Part model, mm, in its own coordinate system. Give positions to 0.01 mm unless a question says otherwise; leave off trailing zeros. Order: outer loops, then holes, each group sorted by start corner. A loop starts at its lowest first (then second) coordinate and runs counter-clockwise, first axis right, second up.
1. Slice it at D-D on x = 0. List the corners of the cut face in (y, z).
2. Slice it at A-A on z = -0.5. List the corners of the cut face in (x, y).
3. Probe line 1 (Z direction, x = -8, y = 4.25); line 2 (X direction, y = -1.5, z = -2.75) (3 decimals); line 3 (X direction, y = 1.75, z = -2). List the from-to ranges inside material, lowest first.
4. Slice it at B-B on z = -6. List the corners of the cut face in (x, y) (3 decimals), and give its area (3 significant figures).
5. Slice it at C-C on y = 4. List the corners of the cut face in (x, z).
6. Drop a flat-ended pin along its axis: pin 1 Ø2 at (y, z) = (4.5, -4.5) entering from +X (3 decimals). Give the stop position or say it passes through.
from build123d import *

# Parameters (mm, degrees)
SKETCH_W               = 37.5
SKETCH_H               = 12
PAD_DEPTH              = 1.4
SKETCH001_W            = 33
SKETCH001_H            = 12
PAD001_DEPTH           = 1.5
SKETCH002_W            = 0.25
SKETCH002_H            = 0.25
PAD002_DEPTH           = 1.5
PAD002_DEPTH_BACK      = 9.5
LINEARPATTERN_COUNT    = 4
LINEARPATTERN_PITCH    = 2.5
PAD003_DEPTH           = 2.25
LINEARPATTERN001_COUNT = 4
LINEARPATTERN001_PITCH = 2.5


with BuildPart() as part:
    # Sketch → Pad (new body)
    with BuildSketch(Plane.XY):
        Rectangle(SKETCH_W, SKETCH_H)
    extrude(amount=PAD_DEPTH)

    # Sketch001 (on Face6 of Pad) → Pad001 (join)
    with BuildSketch(Plane.XY.offset(1.4)):
        with Locations((2.25, 0)):
            Rectangle(SKETCH001_W, SKETCH001_H)
    extrude(amount=PAD001_DEPTH)

    # Sketch002 (on Face5 of Pad001) → Pad002 (join, two sides)
    with BuildSketch(Plane.XY.offset(1.4)) as pad002_sk:
        with Locations((-17.55, -4)):
            Rectangle(SKETCH002_W, SKETCH002_H)
    pad002 = extrude(amount=PAD002_DEPTH) + extrude(pad002_sk.sketch, amount=-PAD002_DEPTH_BACK)

    # LinearPattern: Pad002 ×4
    with Locations(*[(0, i * LINEARPATTERN_PITCH, 0) for i in range(1, LINEARPATTERN_COUNT)]):
        add(pad002)

    # Sketch003 (on Face4 of LinearPattern) → Pad003 (join)
    with BuildSketch(Plane(origin=(0, 0, 0), x_dir=(1, 0, 0), z_dir=(0, 0, -1))):
        Polygon((-18.8, 4.896447), (-18.446447, 5.25), (-16.653553, 5.25), (-16.3, 4.896447), (-16.3, 3.103553), (-16.653553, 2.75), (-18.446447, 2.75), (-18.8, 3.103553), align=None)
    pad003 = extrude(amount=PAD003_DEPTH)

    # LinearPattern001: Pad003 ×4
    with Locations(*[(0, i * LINEARPATTERN001_PITCH, 0) for i in range(1, LINEARPATTERN001_COUNT)]):
        add(pad003)


solid = part.part
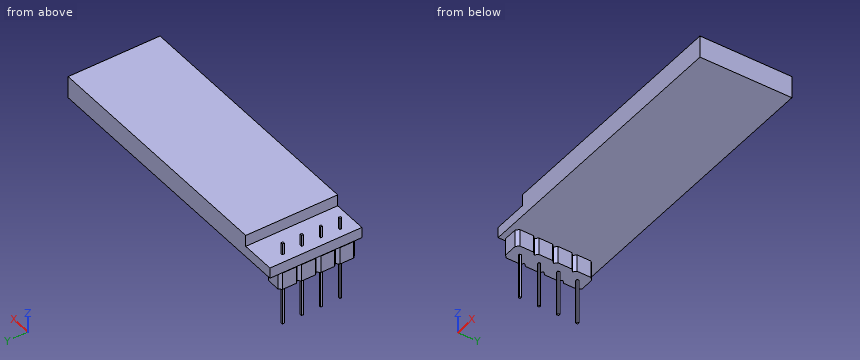
Data:
1. outline: (-6, 0) - (6, 0) - (6, 2.9) - (-6, 2.9) - close
2. outline: (-18.8, -4.9) - (-18.45, -5.25) - (-16.65, -5.25) - (-16.3, -4.9) - (-16.3, -3.1) - (-16.65, -2.75) - (-16.3, -2.4) - (-16.3, -0.6) - (-16.65, -0.25) - (-16.3, 0.1) - (-16.3, 1.9) - (-16.65, 2.25) - (-16.3, 2.6) - (-16.3, 4.4) - (-16.65, 4.75) - (-18.45, 4.75) - (-18.8, 4.4) - (-18.8, 2.6) - (-18.45, 2.25) - (-18.8, 1.9) - (-18.8, 0.1) - (-18.45, -0.25) - (-18.8, -0.6) - (-18.8, -2.4) - (-18.45, -2.75) - (-18.8, -3.1) - close
3. line 1: z = 0 to 2.9
3. line 2: x = -17.675 to -17.425
3. line 3: x = -18.8 to -16.3
4. outline: (-17.675, -4.125) - (-17.425, -4.125) - (-17.425, -3.875) - (-17.675, -3.875) - close; (-17.675, -1.625) - (-17.425, -1.625) - (-17.425, -1.375) - (-17.675, -1.375) - close; (-17.675, 0.875) - (-17.425, 0.875) - (-17.425, 1.125) - (-17.675, 1.125) - close; (-17.675, 3.375) - (-17.425, 3.375) - (-17.425, 3.625) - (-17.675, 3.625) - close
4. area: 0.250 mm2
5. outline: (-18.8, -2.25) - (-16.3, -2.25) - (-16.3, 0) - (18.75, 0) - (18.75, 2.9) - (-14.25, 2.9) - (-14.25, 1.4) - (-18.75, 1.4) - (-18.75, 0) - (-18.8, 0) - close
6. pin 1: stops at x = -17.425
